Input: part model. Units: mm. Frame: model coordinates. Give positions to 0.01 mm unless a question says otherwise; leave off trailing zeros. Loops run counter-clockwise (first coordinate to the right, second up) from the corner with the lowest first, then second, coordinate; pieces in that order, holes last. Notation, with made-up numbers: M -17,38.25 L 29,38.25 A32 cw 29,76.25 Z; hole C 57,-13.5 d2. An arc over 180 degrees is marked long. Return JSON: item names as keys, results as strings. Group by question number.
```python
from build123d import *

# Parameters (mm, degrees)
SKETCH1_R           = 6.35
BOSS_EXTRUDE1_DEPTH = 38.1
CHAMFER1_SIZE       = 2.54
CHAMFER2_SIZE       = 2.54


with BuildPart() as part:
    # Sketch1 → Boss-Extrude1 (new body)
    with BuildSketch(Plane.XY):
        Circle(SKETCH1_R)
    extrude(amount=BOSS_EXTRUDE1_DEPTH)

    # Chamfer1
    chamfer1_edges = [part.edges().sort_by_distance(p)[0] for p in [
        (-6.35, 0, 38.1),
    ]]
    chamfer(chamfer1_edges, length=CHAMFER1_SIZE)

    # Chamfer2
    chamfer2_edges = [part.edges().sort_by_distance(p)[0] for p in [
        (-6.35, 0, 0),
    ]]
    chamfer(chamfer2_edges, length=CHAMFER2_SIZE)


solid = part.part
```
Item 1: Material intervals for line 1 (X direction, y = -1.5, z = 25); line 2 (Z direction, x = -4, y = -4.5); line 3 (X direction, y = -4.25, z = 11), sorted ascending. Write a range as from..to.
Item 2: Section C-C, the plane z = 10. Return loops of the section in (x, y), then the cut area to 3 significant figures.
Item 3: Section A-A, the plane y = 0. Return loops of the section in (x, z), then the cut area to 3 significant figures.
Item 4: First-contact query: pin 1 Ø5 at (x, y) = (-4.5, 3) entering from -Z; pin 2 Ø6 at (x, z) = (-5, 30) entering from +Y; pin 3 Ø4 at (y, z) = (2.5, 6.5) entering from +X; pin 4 Ø5 at (x, z) = (5, 17) entering from -Y. Flat tips, straight axial feed; report the tip coordinate or a pass-through.
Answer below:
{
 "1": {"line 1": "-6.17..6.17", "line 2": "2.21..35.89", "line 3": "-4.72..4.72"},
 "2": {"outline": "C 0,0 d12.7", "area": "127 mm^2"},
 "3": {"outline": "M -6.35,2.54 L -3.81,0 L 3.81,0 L 6.35,2.54 L 6.35,35.56 L 3.81,38.1 L -3.81,38.1 L -6.35,35.56 Z", "area": "471 mm^2"},
 "4": {"pin 1": "z = 0", "pin 2": "y = 6.03", "pin 3": "x = 6.33", "pin 4": "y = -5.84"}
}
